Check sheet for the modelled part. Datum: model origin and axes. Units: mm. Face numbers are marked on the shaded views. A direction names the side the tool comes from. Round coordinates to 2 decimals unless told otherwise and drop trailing zeros. Write each loop counter-clockwise with the first axis right and the second up, starting at its lowest first coordinate (ties: lowest second). Pieces come first, ordered by that corner, then holes. Notation, with made-up numbers: M -2.75,-8.75 L 31.25,-8.75 A23 cw 31.25,9.25 Z; hole C -19.75,84 d2. An arc over 180 degrees is marked long. Answer in a Markdown table with one row per item.
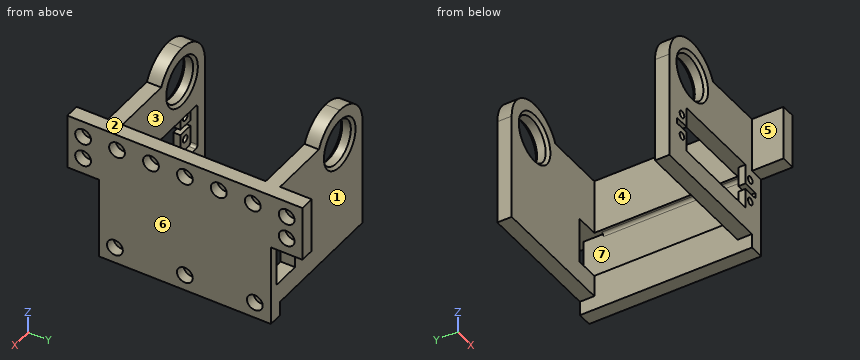
```python
from build123d import *

# Parameters (mm, degrees)
MASS_DEPTH              = 76.2
SKETCH5_R               = 9.652
BEARING_HOLE_DEPTH      = 102.983761741
SKETCH6_W               = 63.5
SKETCH6_H               = 63.5
HOLLOW_DEPTH            = 107.683809823
SKETCH2_R               = 1.5875
SERVO_MOUNT_DEPTH       = 6.35
SERVO_INSET_DEPTH       = 63.5
SERVO_INSET_DEPTH_BACK  = 3.175
SKETCH7_W               = 54.356
SKETCH7_H               = 20.32
BEARING_CHAMFER_SIZE    = 1.27
MINOR_FILLET_R          = 1.27
CUT_EXTRUDE1_DEPTH      = 98.330725666
CUT_EXTRUDE1_DEPTH_BACK = 98.330725666
CUT_EXTRUDE3_DEPTH      = 2.54
CUT_EXTRUDE3_DEPTH_BACK = 98.330725666
SKETCH12_W              = 12.7
SKETCH12_H              = 20.32
SKETCH13_W              = 24.446723308
SKETCH13_H              = 104.14
BOSS_EXTRUDE3_DEPTH     = 6.35
BOSS_EXTRUDE4_DEPTH     = 6.35
SKETCH17_W              = 6.35
SKETCH17_H              = 76.2
BOSS_EXTRUDE5_DEPTH     = 6.35
SKETCH18_R              = 3.5
CUT_EXTRUDE4_DEPTH      = 4.55


with BuildPart() as part:
    # Sketch1 → Mass (new body)
    with BuildSketch(Plane(origin=(0, 0, 0), x_dir=(1, 0, 0), z_dir=(0, 1, 0))):
        with BuildLine():
            Line((-15.270268156, 47.625), (48.229731844, 47.625))
            Line((48.229731844, 47.625), (48.229731844, -9.525))
            Line((48.229731844, -9.525), (0.604731844, -9.525))
            ThreePointArc((0.604731844, -9.525), (-10.620588307, -4.875320151), (-15.270268156, 6.35))
            Line((-15.270268156, 6.35), (-15.270268156, 47.625))
        make_face()
    extrude(amount=MASS_DEPTH)

    # Sketch5 → Bearing Hole (cut, through all)
    with BuildSketch(Plane.XZ):
        with Locations(Location((0.604731844, -6.35, 0), (0, 0, 270))):
            Circle(SKETCH5_R)
    extrude(amount=-BEARING_HOLE_DEPTH, mode=Mode.SUBTRACT)

    # Sketch6 → Hollow (cut, through all)
    with BuildSketch(Plane(origin=(32.780463142, 0, 9.525), x_dir=(-1, 0, 0), z_dir=(0, 0, -1))):
        with Locations((22.650731298, 38.1)):
            Rectangle(SKETCH6_W, SKETCH6_H)
    extrude(amount=HOLLOW_DEPTH, mode=Mode.SUBTRACT)

    # Sketch2 → Servo Mount (cut)
    with BuildSketch(Plane(origin=(0, 6.35, 0), x_dir=(1, 0, 0), z_dir=(0, 1, 0))):
        with Locations(Location((-6.545506188, 39.332658403, 0), (0, 0, 180))):
            Circle(SKETCH2_R)
        with Locations(Location((-6.545506188, 29.162658403, 0), (0, 0, 180))):
            Circle(SKETCH2_R)
        with Locations(Location((40.698493812, 39.332658403, 0), (0, 0, 180))):
            Circle(SKETCH2_R)
        with Locations(Location((40.698493812, 29.162658403, 0), (0, 0, 180))):
            Circle(SKETCH2_R)
        Polygon((-3.243506188, 24.087658403), (37.396493812, 24.087658403), (37.396493812, 32.977658403), (44.254493812, 32.977658403), (44.254493812, 35.517658403), (37.396493812, 35.517658403), (37.396493812, 44.407658403), (-3.243506188, 44.407658403), (-3.243506188, 35.517658403), (-10.101506188, 35.517658403), (-10.101506188, 32.977658403), (-3.243506188, 32.977658403), align=None)
    extrude(amount=-SERVO_MOUNT_DEPTH, mode=Mode.SUBTRACT)

    # Sketch7 → Servo Inset (cut, two sides: drawn at the far end of the back side and taken through both)
    with BuildSketch(Plane(origin=(0, 6.35, 0), x_dir=(1, 0, 0), z_dir=(0, 1, 0)).offset(-SERVO_INSET_DEPTH_BACK)):
        with Locations((17.076493812, 34.247658403)):
            Rectangle(SKETCH7_W, SKETCH7_H)
    extrude(amount=SERVO_INSET_DEPTH + SERVO_INSET_DEPTH_BACK, mode=Mode.SUBTRACT)

    # Bearing Chamfer
    bearing_chamfer_edges = [part.edges().sort_by_distance(p)[0] for p in [
        (0.604731844, 76.2, 3.302),
        (0.604731844, 0, 3.302),
        (0.604731844, 69.85, 3.302),
        (0.604731844, 6.35, 3.302),
    ]]
    chamfer(bearing_chamfer_edges, length=BEARING_CHAMFER_SIZE)

    # Minor fillet
    minor_fillet_edges = [part.edges().sort_by_distance(p)[0] for p in [
        (44.254493812, 36.5125, -44.407658403),
        (44.254493812, 69.85, -34.247658403),
        (44.254493812, 36.5125, -24.087658403),
        (-10.101506188, 4.7625, -24.087658403),
        (-10.101506188, 4.7625, -44.407658403),
    ]]
    fillet(minor_fillet_edges, radius=MINOR_FILLET_R)

    # Sketch9 → Cut-Extrude1 (cut, two sides: drawn at the far end of the back side and taken through both)
    with BuildSketch(Plane(origin=(0, 6.35, 0), x_dir=(1, 0, 0), z_dir=(0, 1, 0)).offset(-CUT_EXTRUDE1_DEPTH_BACK)):
        with BuildLine():
            Line((14.992367963, -0.359064905), (48.229731844, -0.359064905))
            Line((48.229731844, -0.359064905), (48.229731844, -9.525))
            Line((48.229731844, -9.525), (0.604731844, -9.525))
            ThreePointArc((0.604731844, -9.525), (9.134363127, -7.038839202), (14.992367963, -0.359064905))
        make_face()
    extrude(amount=CUT_EXTRUDE1_DEPTH + CUT_EXTRUDE1_DEPTH_BACK, mode=Mode.SUBTRACT)

    # Sketch12 → Cut-Extrude3 (cut, two sides: drawn at the far end of the back side and taken through both)
    with BuildSketch(Plane.XZ.offset(-69.85).offset(-CUT_EXTRUDE3_DEPTH_BACK)):
        with Locations((37.904493812, -34.247658403)):
            Rectangle(SKETCH12_W, SKETCH12_H)
    extrude(amount=CUT_EXTRUDE3_DEPTH + CUT_EXTRUDE3_DEPTH_BACK, mode=Mode.SUBTRACT)

    # Sketch13 → Boss-Extrude3 (add)
    with BuildSketch(Plane.ZY.offset(-41.879731844)):
        with Locations((-11.864296749, 38.1)):
            Rectangle(SKETCH13_W, SKETCH13_H)
    extrude(amount=-BOSS_EXTRUDE3_DEPTH)

    # Sketch16 → Boss-Extrude4 (add)
    with BuildSketch(Plane(origin=(0, 0, -47.625), x_dir=(-1, 0, 0), z_dir=(0, 0, -1))):
        Polygon((-41.879731844, 69.85), (15.270268156, 69.85), (15.270268156, 76.2), (-48.229731844, 76.2), (-48.229731844, 0), (15.270268156, 0), (15.270268156, 6.35), (-41.879731844, 6.35), align=None)
    extrude(amount=BOSS_EXTRUDE4_DEPTH)

    # Sketch17 → Boss-Extrude5 (add)
    with BuildSketch(Plane(origin=(0, 0, -53.975), x_dir=(-1, 0, 0), z_dir=(0, 0, -1))):
        with Locations((-45.054731844, 38.1)):
            Rectangle(SKETCH17_W, SKETCH17_H)
    extrude(amount=BOSS_EXTRUDE5_DEPTH)

    # Sketch18 → Cut-Extrude4 (cut)
    with BuildSketch(Plane(origin=(48.229731844, 0, 0), x_dir=(0, 0, -1), z_dir=(1, 0, 0))):
        with Locations((16.912935095, -6.985)):
            Circle(SKETCH18_R)
        with Locations((6.752935095, -6.985)):
            Circle(SKETCH18_R)
        with Locations((6.752935095, 83.185)):
            Circle(SKETCH18_R)
        with Locations((16.912935095, 83.185)):
            Circle(SKETCH18_R)
        with Locations((53.213, 69.088)):
            Circle(SKETCH18_R)
        with Locations((53.213, 7.112)):
            Circle(SKETCH18_R)
        with Locations((6.752935095, 8.043333333)):
            Circle(SKETCH18_R)
        with Locations((6.752935095, 23.071666667)):
            Circle(SKETCH18_R)
        with Locations((6.752935095, 68.156666667)):
            Circle(SKETCH18_R)
        with Locations((6.752935095, 53.128333333)):
            Circle(SKETCH18_R)
        with Locations((53.213, 38.1)):
            Circle(SKETCH18_R)
        with Locations((6.752935095, 38.1)):
            Circle(SKETCH18_R)
    extrude(amount=-CUT_EXTRUDE4_DEPTH, mode=Mode.SUBTRACT)


solid = part.part
```
1. Go/stop test with flat-tipped pins: pin 1 (3.5 mm diameter, centred on y = 82, z = -16.5, fed in from +X); pin 2 (4 mm diameter, centred on y = 0.5, z = -6, fed in from -X); pin 3 (1 mm diameter, centred on x = -6.5, y = 1.5, fed in from -Z) (3 decimals); pin 4 (2.5 mm diameter, centred on x = 42.5, y = 1.5, fed in from +Z). Record where each tip stops, or that it passes through.
Found:
| item | result |
|---|---|
| pin 1 | stops at x = 43.68 |
| pin 2 | stops at x = -15.27 |
| pin 3 | stops at z = -53.975 |
| pin 4 | stops at z = 0.36 |
2. Section check A-A, the plane x = 24. Record the cut outline in (y, z) (3 decimals).
Found:
| item | result |
|---|---|
| outline | M 0,-53.975 L 6.35,-53.975 L 6.35,-44.408 L 0,-44.408 Z; M 0,-24.088 L 6.35,-24.088 L 6.35,0.359 L 0,0.359 Z; M 69.85,-53.975 L 76.2,-53.975 L 76.2,0.359 L 69.85,0.359 Z |
3. Scan lines: L1, parallel to Z at x = 47, y = 38 (1 decimal); L2, parallel to Y at x = 4.5, z = -45.5; L3, parallel to Y at x = 45.5, z = -53.5. Record each from-to range of solid material in increasing order.
Found:
| item | result |
|---|---|
| L1 | z = -60.3 to -56.7, -49.7 to -10.3, -3.3 to 0.4 |
| L2 | y = 0 to 6.35, 69.85 to 76.2 |
| L3 | y = 0 to 3.62, 10.6 to 34.61, 41.59 to 65.6, 72.58 to 76.2 |
4. Section check C-C, the plane x = 7.5. Count the separate pieces of the cut face and the enclosed holes in it, and give its area (3 significant figures).
Found:
| item | result |
|---|---|
| separate pieces | 5 |
| enclosed holes | 0 |
| area | 477 mm2 |
5. Access from +Z, -Z, +X, -X, +Y, -Y to the whole of each face (thin tool, end or side, straight path). Record for the marked faces 4, 5, 6 and 7.
Found:
| item | result |
|---|---|
| face 4 | +Z, -Z, -X |
| face 5 | +Z, -Z, -X, -Y |
| face 6 | +Z, -Z, +X, +Y, -Y |
| face 7 | +Y |
6. Section check B-B, the plane y = 38.1. Record the cut outline in (x, z) (1 decimal).
Found:
| item | result |
|---|---|
| outline | M 41.9,-60.3 L 48.2,-60.3 L 48.2,-56.7 L 43.7,-56.7 L 43.7,-49.7 L 48.2,-49.7 L 48.2,-10.3 L 43.7,-10.3 L 43.7,-3.3 L 48.2,-3.3 L 48.2,0.4 L 41.9,0.4 L 41.9,-24.1 L 43,-24.1 A1.3 cw 44.3,-25.4 L 44.3,-43.1 A1.3 cw 43,-44.4 L 41.9,-44.4 Z |
7. Draft check along Y on the marked faces 1, 2 and 3. Enter one of: +Y half, -Y half, draft (parallel to the pull), parting line (faces both ways), or undercut.
Found:
| item | result |
|---|---|
| face 1 | +Y half |
| face 2 | draft |
| face 3 | undercut |
